Autodesk Inventor part; units mm, degrees
ref_plane "YZ Plane" through (0, 0, 0) normal (1, 0, 0) x (0, 1, 0)
ref_plane "XZ Plane" through (0, 0, 0) normal (0, 1, 0) x (-1, 0, 0)
ref_plane "XY Plane" through (0, 0, 0) normal (0, 0, 1) x (1, 0, 0)
sketch "スケッチ1" plane through (0, 0, 0) normal (0, 0, 1) x (1, 0, 0)
  line L0 (7.5, -7.5) -> (-7.5, -7.5)
  line L1 (-7.5, -7.5) -> (-7.5, 7.5)
  line L2 (-7.5, 7.5) -> (7.5, 7.5)
  line L3 (7.5, 7.5) -> (7.5, -7.5)
  line L4 (7.5, -7.5) -> (-7.5, 7.5) construction
  line L5 (-7.5, -7.5) -> (7.5, 7.5) construction
  point P0 (0, 0)
  dimension "d0" = 15
  dimension "d1" = 15
extrude "押し出し1" add sketch "スケッチ1" along normal blind 280
shell "シェル1" thickness 1 removed faces 2 at (2.5, -2.5, 0) at (2.5, -2.5, 280)
sketch "スケッチ2" plane through (-7.5, 7.5, 0) normal (0, 1, 0) x (1, 0, 0)
  line L0 (7.5, -172.043) -> (7.5, -107.957) construction
  line L1 (15, -280) -> (0, -280)
  line L2 (0, 0) -> (0, -280)
  line L3 (0, -140) -> (7.5, -140) construction
  point P0 (7.5, 0)
  point P1 (7.5, -280)
  point P2 (7.5, -272)
  point P3 (7.5, -8)
  dimension "d5" = 64.086
  dimension "d29" = 264
hole "穴1" at (0, 7.5, 172.043) at (0, 7.5, 107.957) at (0, 7.5, 272) at (0, 7.5, 8) direction (0, -1, 0) diameter 3.2 end through all
sketch "スケッチ3" plane through (-7.5, -7.5, 0) normal (-1, 0, 0) x (0, 0, 1)
  line L0 (20, 7.5) -> (260, 7.5)
  line L1 (0, 15) -> (280, 15)
  line L2 (280, 15) -> (280, 0)
  point P0 (0, 7.5)
  point P1 (140, 7.5)
  point P2 (140, 15)
  point P3 (280, 7.5)
  dimension "d13" = 240
hole "穴2" at (-7.5, 0, 260) at (-7.5, 0, 20) direction (1, 0, 0) diameter 10 end through all
properties part number "BaseSlideSTOPPERsq2"
The model under review builds one solid part; all positions refer to its coordinate system, in mm. A direction names the side the tool comes from. Round coordinates to 2 decimals unless told otherwise and drop trailing zeros. Loops run counter-clockwise (first coordinate to the right, second up) from the corner with the lowest first, then second, coordinate; pieces in that order, holes last. Notation, with made-up numbers: M 67,79 L 90,79 A20 cw 90,102 Z; hole C 49.25,87.25 d1. An arc over 180 degrees is marked long. Answer as CSV lines item,"result".
1. To check wall thickness, follow L1, parallel to Z at x = 6.7, y = 0; L2, parallel to Z at x = 0, y = 7.2; L3, parallel to Y at x = -1.75, z = 163. State the ranges of each line that lie inside material, in increasing order. Write a range as [from, to].
Outcome:
L1,"z = [0, 15], [25, 255], [265, 280]"
L2,"z = [0, 6.4], [9.6, 106.36], [109.56, 170.44], [173.64, 270.4], [273.6, 280]"
L3,"y = [-7.5, -6.5], [6.5, 7.5]"
2. We need section C-C (z = 116). Give the boundary of the cut face in (x, y).
Outcome:
outline,"M -7.5,-7.5 L 7.5,-7.5 L 7.5,7.5 L -7.5,7.5 Z; hole M -6.5,-6.5 L 6.5,-6.5 L 6.5,6.5 L -6.5,6.5 Z"
3. We need section A-A (x = 4). Give the boundary of the cut face in (y, z), plus the area to 3 significant figures.
Outcome:
outline,"M -7.5,0 L -6.5,0 L -6.5,280 L -7.5,280 Z; M 6.5,0 L 7.5,0 L 7.5,280 L 6.5,280 Z"
area,"560 mm2"
4. We need section B-B (y = 0). Give the boundary of the cut face in (x, z), plus the area to 3 significant figures.
Outcome:
outline,"M -7.5,0 L -6.5,0 L -6.5,15 L -7.5,15 Z; M -7.5,25 L -6.5,25 L -6.5,255 L -7.5,255 Z; M -7.5,265 L -6.5,265 L -6.5,280 L -7.5,280 Z; M 6.5,0 L 7.5,0 L 7.5,15 L 6.5,15 Z; M 6.5,25 L 7.5,25 L 7.5,255 L 6.5,255 Z; M 6.5,265 L 7.5,265 L 7.5,280 L 6.5,280 Z"
area,"520 mm2"
5. For faces 1 (the face through (-7, 0, 15)), 2 (the face through (6.5, 0, 138)), list the 3-axis set-ups (+Z, -Z, +X, -X, +Y, -Y) from which the entire face can be reached by the end or side of a thin tool; tool diameter is ignored.
Outcome:
face 1,"+X, -X"
face 2,"+Z, -Z"
6. Draft analysis for pull direction Z (two halves, no side actions). For faces 3 (the face through (-7, 0, 280)), 4 (the face through (7, 0, 15)), 5 (the face through (-6.99, -1.5, 264.77)), 6 (the face through (7.5, 0, 138)), state which applies: pulls with the +Z half, pulls with the -Z half, needs draft (parallel to the pull), parting line crosses it, or undercut.
Outcome:
face 3,"pulls with the +Z half"
face 4,"undercut"
face 5,"undercut"
face 6,"needs draft"
7. Insertion check: pin 1 Ø9 at (y, z) = (0, 260) entering from -X. The pin has a flat end and moves straight along its axis. Give the tip position at first contact, or say it passes through.
Outcome:
pin 1,"passes through"
